from build123d import *

# Parameters (mm, degrees)
BOSS_EXTRUDE1_DEPTH = 12
SKETCH2_OUTSIDE_W   = 77.868
SKETCH2_OUTSIDE_H   = 81.89
SKETCH2_OUTSIDE_R   = 13
CUT_EXTRUDE2_DEPTH  = 12
CUT_EXTRUDE2_DRAFT  = -60
SKETCH3_R           = 10
BOSS_EXTRUDE2_DEPTH = 75
CHAMFER1_SIZE       = 1


with BuildPart() as part:
    # Sketch1 → Boss-Extrude1 (new body)
    with BuildSketch(Plane(origin=(0, 0, 0), x_dir=(1, 0, 0), z_dir=(0, 1, 0))):
        Polygon((13, 7.505553499), (0, 15.011106999), (-13, 7.505553499), (-13, -7.505553499), (0, -15.011106999), (13, -7.505553499), align=None)
    extrude(amount=BOSS_EXTRUDE1_DEPTH)


with BuildPart() as cut_extrude2_tool:
    # Sketch2 outside → Cut-Extrude2 (with draft: the straight prism first)
    with BuildSketch(Plane(origin=(0, 12, 0), x_dir=(1, 0, 0), z_dir=(0, 1, 0))):
        Rectangle(SKETCH2_OUTSIDE_W, SKETCH2_OUTSIDE_H)
        Circle(SKETCH2_OUTSIDE_R, mode=Mode.SUBTRACT)
    extrude(amount=-CUT_EXTRUDE2_DEPTH)
    # Cut-Extrude2: the draft: its side faces are tilted about the plane it starts from
    cut_extrude2_sides = [cut_extrude2_tool.faces().sort_by_distance(p)[0] for p in [
        (0, 6, 40.945),
        (38.934, 6, 0),
        (0, 6, -40.945),
        (-38.934, 6, 0),
        (-13, 6, 0),
    ]]
    draft(cut_extrude2_sides, Plane(origin=(0, 12, 0), x_dir=(1, 0, 0), z_dir=(0, 1, 0)), CUT_EXTRUDE2_DRAFT)


with BuildPart() as part_1:
    add(part.part)

    # Cut-Extrude2: cut by cut_extrude2_tool
    add(cut_extrude2_tool.part, mode=Mode.SUBTRACT)

    # Sketch3 → Boss-Extrude2 (add)
    with BuildSketch(Plane.XZ):
        with Locations(Location((0, 0, 0), (0, 0, 90))):
            Circle(SKETCH3_R)
    extrude(amount=BOSS_EXTRUDE2_DEPTH)

    # Chamfer1
    chamfer1_edges = [part_1.edges().sort_by_distance(p)[0] for p in [
        (0, -75, -10),
    ]]
    chamfer(chamfer1_edges, length=CHAMFER1_SIZE)


solid = part_1.part
Work out the finished part from the listing and answer in its coordinate system (mm). A direction names the side the tool comes from. Give positions to 0.01 mm unless a question says otherwise; leave off trailing zeros. Loops run counter-clockwise (first coordinate to the right, second up) from the corner with the lowest first, then second, coordinate; pieces in that order, holes last. Notation, with made-up numbers: (-12.5, 13.25) -> (6.5, 13.25) arc R22 ccw to (6.5, 48.25) -> close; hole circle Ø2 at (-32, 72.5). An arc over 180 degrees is marked (long way). Use a Markdown table: item, result. Add a question column.
1) Consider line 1 along Y through (x, z) = (-11.75, -4); line 2 along X through (y, z) = (-33.5, -0.5); line 3 along Y through (x, z) = (-7.5, -6.5). Determine where each line is inside the solid, lowest interval first.
2) The part is cut by section A-A, the plane y = -22. Determine the outline of the cut face in (x, z), plus the area to 3 significant figures.
3) Which of the six approach directions +Z, -Z, +X, -X, +Y, -Y give full straight-line access (tool end or side, diameter ignored) to faces 1 (the flat face through (13, 6, 0)), 2 (the flat face through (-5, 0, -9))?
4) Each of these flat-tipped pins is pushed along its axis until it touches: P1, Ø12, axis at y = -43.5, z = -9, coming from the -X side; P2, Ø8, axis at y = -27, z = 11.5, coming from the -X side; P3, Ø1, axis at x = 5.5, y = -42, coming from the -Z side. Where does it stop, or does it pass through?
Reported:
| question | item | result |
|---|---|---|
| 1 | line 1 | y = 0 to 12 |
| 1 | line 2 | x = -9.99 to 9.99 |
| 1 | line 3 | y = -74.08 to 12 |
| 2 | outline | circle Ø20 at (0, 0) |
| 2 | area | 314 mm^2 |
| 3 | face 1 | +Z, -Z, +X, +Y, -Y |
| 3 | face 2 | -Y |
| 4 | P1 | stops at x = -9.54 |
| 4 | P2 | stops at x = -6.61 |
| 4 | P3 | stops at z = -8.66 |
